Can you work these out from the model? Positions are in its coordinate system, mm. A direction names the side the tool comes from. Round coordinates to 2 decimals unless told otherwise and drop trailing zeros. Loops run counter-clockwise (first coordinate to the right, second up) from the corner with the lowest first, then second, coordinate; pieces in that order, holes last. Notation, with made-up numbers: (-21, 38.25) -> (7, 38.25) arc R22 cw to (7, 45.25) -> close; hole circle Ø1 at (81.5, 19.5). An arc over 180 degrees is marked (long way). Answer as a JSON object with one key per item and string values.
```python
from build123d import *

# Parameters (mm, degrees)
F1_DEPTH = 1


with BuildPart() as f1:
    # F0 (on Front) → F1 (new body, symmetric)
    with BuildSketch(Plane.XZ):
        with BuildLine():
            Line((78.5832557587, 72), (-81, 72))
            Line((-81, 72), (-81, -72))
            Line((-81, -72), (-2.5758354459, -72))
            Line((-2.5758354459, -72), (-2.5758354459, 0))
            Line((-2.5758354459, 0), (-0.5758354459, 0))
            Line((-0.5758354459, 0), (-0.5758354459, -72))
            Line((-0.5758354459, -72), (70.0140722752, -72))
            ThreePointArc((70.0140722752, -72), (80.6669131732, -73.9550899306), (89.9312699398, -79.5655346133))
            add(Edge.make_bspline(
                [(81, -72), (84.4635983749, -74.8141629135), (87.3994420895, -77.31779147), (89.9312699398, -79.5655346133)],
                knots=[0, 0, 0, 0, 0.0519635784, 0.0519635784, 0.0519635784, 0.0519635784], degree=3))
            Line((81, -72), (81, 71.8534467353))
            ThreePointArc((81, 71.8534467353), (79.7938476168, 71.9633280631), (78.5832557587, 72))
        make_face()
        with BuildLine():
            Line((81, 72), (81, 71.8534467353))
            Line((81, 71.8534467353), (81, -72))
            add(Edge.make_bspline(
                [(81, -72), (84.4635983749, -74.8141629135), (87.3994420895, -77.31779147), (89.9312699398, -79.5655346133)],
                knots=[0, 0, 0, 0, 0.0519635784, 0.0519635784, 0.0519635784, 0.0519635784], degree=3))
            add(Edge.make_bspline(
                [(89.9312699398, -79.5655346133), (102.3651827748, -90.6042955291), (108.3217609729, -101.383114475), (158.7265599507, -121.9444495797), (190.0937696642, -109.2006741806), (218.0848423474, -98.6219057368)],
                knots=[0.0519635784, 0.0519635784, 0.0519635784, 0.0519635784, 0.3071588928, 0.6171111846, 1, 1, 1, 1], degree=3))
            Line((218.0848423474, -98.6219057368), (229.9621609222, -94.0626303033))
            Line((229.9621609222, -94.0626303033), (212.9396833188, -49.7175600446))
            Line((212.9396833188, -49.7175600446), (214.8068441718, -49.0008241456))
            Line((214.8068441718, -49.0008241456), (231.8293217752, -93.3458944042))
            Line((231.8293217752, -93.3458944042), (246.0922551423, -87.8708672505))
            Line((246.0922551423, -87.8708672505), (212.0472999355, 0.8192732668))
            Line((212.0472999355, 0.8192732668), (188.707789273, -8.1399254719))
            add(Edge.make_bspline(
                [(83.8849046159, 71.2845150158), (105.3400246798, 65.3861290478), (124.0549392531, 35.6814961762), (138.1532322102, 1.7025226497), (170.7937318796, -14.1268512491), (188.707789273, -8.1399254719)],
                knots=[0.0153089318, 0.0153089318, 0.0153089318, 0.0153089318, 0.3648606153, 0.6619581151, 1, 1, 1, 1], degree=3))
            add(Edge.make_bspline(
                [(81, 72), (81.9838635002, 71.7816800805), (82.9452582497, 71.542840158), (83.8849046159, 71.2845150158)],
                knots=[0, 0, 0, 0, 0.0153089318, 0.0153089318, 0.0153089318, 0.0153089318], degree=3))
        make_face()
        with BuildLine():
            ThreePointArc((83.8849046159, 71.2845150158), (82.45292226, 71.6220712762), (81, 71.8534467353))
            Line((81, 71.8534467353), (81, 72))
            add(Edge.make_bspline(
                [(81, 72), (81.9838635002, 71.7816800805), (82.9452582497, 71.542840158), (83.8849046159, 71.2845150158)],
                knots=[0, 0, 0, 0, 0.0153089318, 0.0153089318, 0.0153089318, 0.0153089318], degree=3))
        make_face(mode=Mode.SUBTRACT)
    extrude(amount=F1_DEPTH, both=True)


solid = f1.part
```
Q1. On a 3-axis mill with a long thin cutter (end or side, diameter ignored), from which of +Z, -Z, +X, -X, +Y, -Y can I reach the whole of each face in a straight line? I mean faces 1 (the flat face through (44, -1, -24)), 2 (the flat face through (221.57, -0.01, -72.2)), 3 (the flat face through (200.54, -0.01, -3.6)). Say none if no direction works.
Determined:
{"face 1": "+Z, -Z, +X, -X, -Y", "face 2": "+Y, -Y", "face 3": "+Z, +Y, -Y"}
Q2. We'd pull the mould along Z, two halves only. Please class faces 4 (the flat face through (44, 1, -24)), 5 (the flat face through (223.199, -0.014, -70.863)), 6 (the cylindrical face through (80.52, -0.01, -73.9)): pulls with the +Z half, pulls with the -Z half, needs draft (parallel to the pull), parting line crosses it, or undercut.
Determined:
{"face 4": "needs draft", "face 5": "undercut", "face 6": "pulls with the -Z half"}
Q3. I'm going to push a flat-ended pin straight in: pin 1 (1 mm diameter, centred on y = -0.5, z = -39, fed in from +X). Where does the tip first touch, or does it pass through?
Determined:
{"pin 1": "x = 227.52"}
Q4. I want a section at B-B, the plane x = 32.5. Write out the boundary of the cut face in (y, z), then the cut area to 3 significant figures.
Determined:
{"outline": "(-1, -72) -> (1, -72) -> (1, 72) -> (-1, 72) -> close", "area": "288 mm²"}
Q5. If I drill on L1, parallel to X at y = -0.05, z = -53; L2, parallel to Z at x = 61.5, y = 0.55; L3, parallel to X at y = -0.7, z = -81.5, over which ranges is the centre line in solid material (lowest first)? Write a range as [from, to].
Determined:
{"L1": "[-81, -2.58], [-0.58, 214.2], [216.34, 232.71]", "L2": "[-72, 72]", "L3": "[92.08, 225.14], [227.28, 243.65]"}
Q6. I want a section at A-A, the plane x = 222. Write out the boundary of the cut face in (y, z), then the cut area to 3 significant figures.
Determined:
{"outline": "(-1, -97.12) -> (1, -97.12) -> (1, -73.32) -> (-1, -73.32) -> close; (-1, -67.74) -> (1, -67.74) -> (1, -25.11) -> (-1, -25.11) -> close", "area": "133 mm²"}
